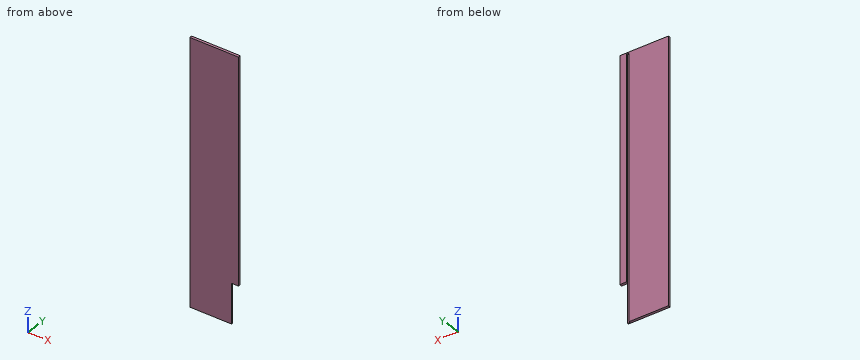
```python
from build123d import *

# Parameters (mm, degrees)
F0_W     = 350
F0_H     = 1885
F1_DEPTH = 18
F2_W     = 50
F2_H     = 285
F3_DEPTH = 18
F4_W     = 18
F4_H     = 1876
F5_DEPTH = 9


with BuildPart() as f1:
    # F0 (on Front) → F1 (new body)
    with BuildSketch(Plane.XZ):
        Rectangle(F0_W, F0_H)
    extrude(amount=F1_DEPTH)

    # F2 (on face) → F3 (cut)
    with BuildSketch(Plane.XZ.offset(18)):
        with Locations((150, -800)):
            Rectangle(F2_W, F2_H)
    extrude(amount=-F3_DEPTH, mode=Mode.SUBTRACT)

    # F4 (on face) → F5 (cut)
    with BuildSketch(Plane(origin=(0, 0, 0), x_dir=(-1, 0, 0), z_dir=(0, 1, 0))):
        with Locations((-116, -4.5)):
            Rectangle(F4_W, F4_H)
    extrude(amount=-F5_DEPTH, mode=Mode.SUBTRACT)


solid = f1.part
```
Geometry: final body of the model. Coordinates: model frame, mm. Coordinates: 2 decimals unless noted, no trailing zeros. Order: outer loops, then holes, each group sorted by start corner. A loop starts at its lowest first (then second) coordinate and runs counter-clockwise, first axis right, second up. Notation, with made-up numbers: M 66,-22 L 92,-22 A14 cw 92,-11 Z; hole C -5,-20.75 d4. An arc over 180 degrees is marked long. Answer in a Markdown table with one row per item. Add a question column.
Q1. Line query: L1, parallel to X at y = -3, z = 423; L2, parallel to Y at x = 108, z = -510.5; L3, parallel to X at y = -10.25, z = -665. Output: solid intervals per line, ascending.
Q2. Contact query for flat-ended pins moving along their axis: P1, Ø9, axis at x = 158.5, y = -5, coming from the -Z side; P2, Ø9, axis at x = 113, z = 323, coming from the +Y side; P3, Ø2.5, axis at x = 111.5, y = -4, coming from the -Z side. Output: stop coordinate, or through.
Q3. Section query C-C on z = -731.5. Return the cut outline in (x, y).
Q4. Section query B-B on z = 143. Return the cut outline in (x, y).
Q5. Section query A-A on y = -6.25. Return the cut outline in (x, z), and give its area (3 significant figures).
Completed:
| question | item | result |
|---|---|---|
| 1 | L1 | x = -175 to 107, 125 to 175 |
| 1 | L2 | y = -18 to -9 |
| 1 | L3 | x = -175 to 125 |
| 2 | P1 | stops at z = -657.5 |
| 2 | P2 | stops at y = -9 |
| 2 | P3 | stops at z = 933.5 |
| 3 | outline | M -175,-18 L 125,-18 L 125,-9 L 107,-9 L 107,0 L -175,0 Z |
| 4 | outline | M -175,-18 L 175,-18 L 175,0 L 125,0 L 125,-9 L 107,-9 L 107,0 L -175,0 Z |
| 5 | outline | M -175,-942.5 L 107,-942.5 L 107,933.5 L 125,933.5 L 125,-657.5 L 175,-657.5 L 175,942.5 L -175,942.5 Z |
| 5 | area | 612,000 mm2 |
